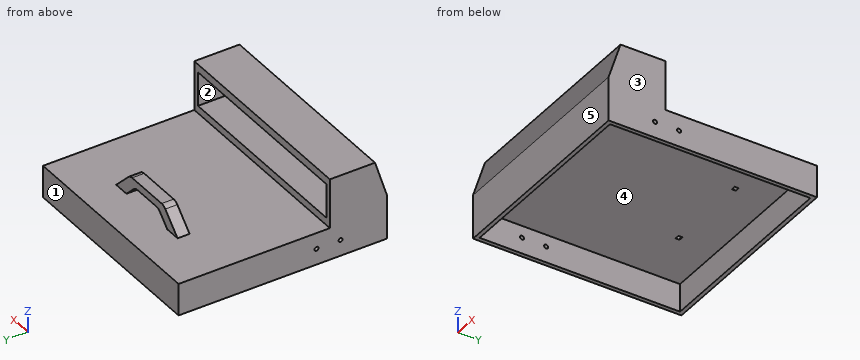
from build123d import *

# Parameters (mm, degrees)
SKETCH1_W           = 330.2
SKETCH1_H           = 330.2
BOSS_EXTRUDE1_DEPTH = 50.8
BOSS_EXTRUDE2_START = 254
BOSS_EXTRUDE2_DEPTH = 19.05
SHELL1_START        = 6.35
SHELL1_OUTLINE_W    = 317.5
SHELL1_OUTLINE_H    = 44.45
SHELL1_DEPTH        = 317.5
SHELL1_START_2      = 260.35
SHELL1_2_DEPTH      = 6.35
SKETCH3_R           = 3.175
CUT_EXTRUDE1_DEPTH  = 475.544431862
BOSS_EXTRUDE3_DEPTH = 330.2
SKETCH5_W           = 312.91275174
SKETCH5_H           = 54.204225569
CUT_EXTRUDE2_DEPTH  = 68.58


# Read off the part's stored shape, not the designer's step: Shell1
with BuildPart() as part:
    # Sketch1 → Boss-Extrude1 (new body)
    with BuildSketch(Plane.XY):
        with Locations((165.1, 165.1)):
            Rectangle(SKETCH1_W, SKETCH1_H)
    extrude(amount=BOSS_EXTRUDE1_DEPTH)

    # Sketch2 → Boss-Extrude2 (add)
    with BuildSketch(Plane(origin=(0, 0, 0), x_dir=(1, 0, 0), z_dir=(0, 1, 0)).offset(BOSS_EXTRUDE2_START)):
        with BuildLine():
            Line((142.104085231, -72.303901903), (188.095914769, -72.303901903))
            ThreePointArc((188.095914769, -72.303901903), (192.95599436, -71.337171966), (197.07617089, -68.584158024))
            Line((197.07617089, -68.584158024), (214.860328914, -50.8))
            Line((214.860328914, -50.8), (239.897502761, -50.8))
            Line((239.897502761, -50.8), (209.987762385, -80.709740376))
            ThreePointArc((209.987762385, -80.709740376), (205.867585855, -83.462754317), (201.007506264, -84.429484254))
            Line((201.007506264, -84.429484254), (129.192493736, -84.429484254))
            ThreePointArc((129.192493736, -84.429484254), (124.332414145, -83.462754317), (120.212237615, -80.709740376))
            Line((120.212237615, -80.709740376), (90.302497239, -50.8))
            Line((90.302497239, -50.8), (115.339671086, -50.8))
            Line((115.339671086, -50.8), (133.12382911, -68.584158024))
            ThreePointArc((133.12382911, -68.584158024), (137.24400564, -71.337171966), (142.104085231, -72.303901903))
        make_face()
    extrude(amount=BOSS_EXTRUDE2_DEPTH)

    # Shell1 outline → Shell1 (cut)
    with BuildSketch(Plane(origin=(0, 0, 0), x_dir=(1, 0, 0), z_dir=(0, 1, 0)).offset(SHELL1_START)):
        with Locations((165.1, -22.225)):
            Rectangle(SHELL1_OUTLINE_W, SHELL1_OUTLINE_H)
    extrude(amount=SHELL1_DEPTH, mode=Mode.SUBTRACT)

    # Shell1 2 outline → Shell1 2 (cut)
    with BuildSketch(Plane(origin=(0, 0, 0), x_dir=(1, 0, 0), z_dir=(0, 1, 0)).offset(SHELL1_START_2)):
        with BuildLine():
            Line((192.738689455, -78.079484254), (201.007506264, -78.079484254))
            ThreePointArc((201.007506264, -78.079484254), (203.43754606, -77.596119286), (205.497634325, -76.219612315))
            Line((205.497634325, -76.219612315), (237.26724664, -44.45))
            Line((237.26724664, -44.45), (230.190585035, -44.45))
            Line((230.190585035, -44.45), (201.56629895, -73.074286085))
            ThreePointArc((201.56629895, -73.074286085), (197.491905042, -76.1755001), (192.738689455, -78.079484254))
        make_face()
        with BuildLine():
            Line((128.63370105, -73.074286085), (100.009414965, -44.45))
            Line((100.009414965, -44.45), (92.93275336, -44.45))
            Line((92.93275336, -44.45), (124.702365675, -76.219612315))
            ThreePointArc((124.702365675, -76.219612315), (126.76245394, -77.596119286), (129.192493736, -78.079484254))
            Line((129.192493736, -78.079484254), (137.461310545, -78.079484254))
            ThreePointArc((137.461310545, -78.079484254), (132.708094958, -76.1755001), (128.63370105, -73.074286085))
        make_face()
    extrude(amount=SHELL1_2_DEPTH, mode=Mode.SUBTRACT)

    # Sketch3 → Cut-Extrude1 (cut, through all)
    with BuildSketch(Plane.ZY):
        with Locations((25.4, 111.6816843)):
            Circle(SKETCH3_R)
        with Locations((25.4, 73.5816843)):
            Circle(SKETCH3_R)
    extrude(amount=-CUT_EXTRUDE1_DEPTH, mode=Mode.SUBTRACT)

    # Sketch4 → Boss-Extrude3 (add)
    with BuildSketch(Plane.ZY):
        Polygon((50.8, 0), (69.908855574, 0), (129.44460093, 18.967737852), (129.44460093, 90.50525308), (50.8, 90.50525308), align=None)
    extrude(amount=-BOSS_EXTRUDE3_DEPTH)

    # Sketch5 → Cut-Extrude2 (cut)
    with BuildSketch(Plane(origin=(0, 90.50525308, 0), x_dir=(1, 0, 0), z_dir=(0, 1, 0))):
        with Locations((164.794269249, -89.730963472)):
            Rectangle(SKETCH5_W, SKETCH5_H)
    extrude(amount=-CUT_EXTRUDE2_DEPTH, mode=Mode.SUBTRACT)


solid = part.part
Source: CAD feature listing. Evaluate the final solid. Frame: model axes, mm. Face numbers are marked on the shaded views. A direction names the side the tool comes from. Round coordinates to 2 decimals unless told otherwise and drop trailing zeros. Loops run counter-clockwise (first coordinate to the right, second up) from the corner with the lowest first, then second, coordinate; pieces in that order, holes last. Notation, with made-up numbers: M 20.25,-30 L 33.25,-30 A37 ccw 33.25,8 Z; hole C 44,54.5 d3. An arc over 180 degrees is marked long. Return JSON: item names as keys, results as strings. Group by question number.
1. Section query C-C on x = 23. Output: boundary loops of the cut face in (y, z), and give its area (3 significant figures).
2. Section query A-A on x = 159. Output: boundary loops of the cut face in (y, z), and give its area (3 significant figures).
3. Reachability of the marked faces 4 and 5 from +Z, -Z, +X, -X, +Y, -Y: full face, straight path, thin tool, end or side. Return the list, or none.
4. Material intervals for line 1 along Y through (x, z) = (1.5, 25.4); line 2 along Y through (x, z) = (1, 25); line 3 along Y through (x, z) = (158.5, 35.5), sorted ascending. Write a range as from..to.
5. Section query D-D on x = 109. Output: boundary loops of the cut face in (y, z).
6. Mould query, pull axis X, two halves, no side actions, for the marked faces 1, 2 and 3. Classes: released by +X, released by -X, zero draft, split by the parting line, or undercut.
7. Pin query (flat end, axial travel): pin 1 (17 mm diameter, centred on x = 106, z = 67.5, fed in from +Y); pin 2 (8 mm diameter, centred on x = 79.5, y = 226.5, fed in from +Z); pin 3 (8 mm diameter, centred on x = 196.5, y = 222.5, fed in from -Z). Return the tip coordinate at first contact, or that it passes through.
8. Section query B-B on z = 11.5. Output: boundary loops of the cut face in (x, y).
Checks:
{
 "1": {"outline": "M 0,0 L 6.35,0 L 6.35,44.45 L 323.85,44.45 L 323.85,0 L 330.2,0 L 330.2,50.8 L 90.51,50.8 L 90.51,62.63 L 21.93,62.63 L 21.93,116.83 L 90.51,116.83 L 90.51,129.44 L 18.97,129.44 L 0,69.91 Z", "area": "5,500 mm²"},
 "2": {"outline": "M 0,0 L 6.35,0 L 6.35,44.45 L 323.85,44.45 L 323.85,0 L 330.2,0 L 330.2,50.8 L 90.51,50.8 L 90.51,62.63 L 21.93,62.63 L 21.93,116.83 L 90.51,116.83 L 90.51,129.44 L 18.97,129.44 L 0,69.91 Z; M 254,72.3 L 273.05,72.3 L 273.05,84.43 L 254,84.43 Z", "area": "5,730 mm²"},
 "3": {"face 4": "-Z", "face 5": "+Z, -Z, +X, -X, -Y"},
 "4": {"line 1": "y = 0..70.41, 76.76..108.51, 114.86..330.2", "line 2": "y = 0..70.43, 76.73..108.53, 114.83..330.2", "line 3": "y = 0..6.35, 323.85..330.2"},
 "5": {"outline": "M 0,0 L 6.35,0 L 6.35,44.45 L 323.85,44.45 L 323.85,0 L 330.2,0 L 330.2,50.8 L 273.05,50.8 L 273.05,69.5 L 254,69.5 L 254,50.8 L 90.51,50.8 L 90.51,62.63 L 21.93,62.63 L 21.93,116.83 L 90.51,116.83 L 90.51,129.44 L 18.97,129.44 L 0,69.91 Z; hole M 260.35,53.44 L 266.7,53.44 L 266.7,60.52 L 260.35,60.52 Z"},
 "6": {"face 1": "zero draft", "face 2": "undercut", "face 3": "released by +X"},
 "7": {"pin 1": "stops at y = 273.05", "pin 2": "stops at z = 50.8", "pin 3": "stops at z = 44.45"},
 "8": {"outline": "M 0,0 L 330.2,0 L 330.2,330.2 L 0,330.2 Z; hole M 6.35,6.35 L 323.85,6.35 L 323.85,323.85 L 6.35,323.85 Z"}
}
